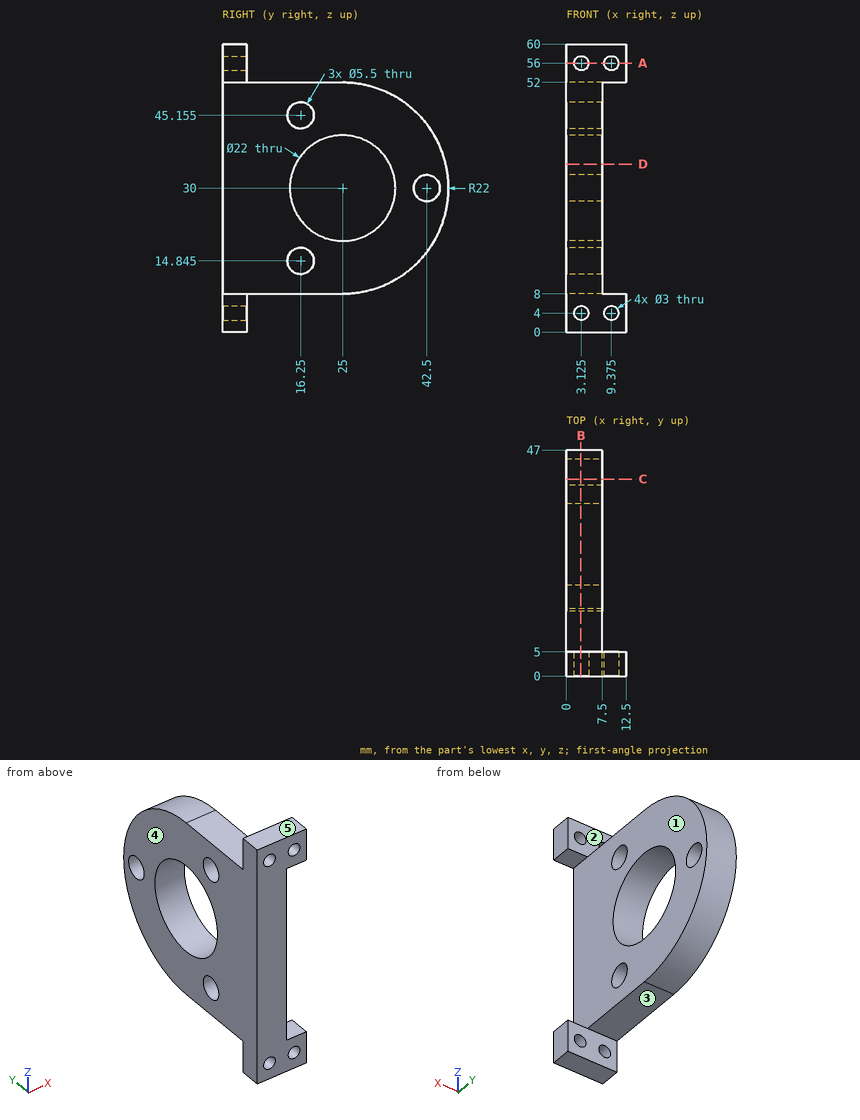
For this review, use the dimensioned drawing (mm, ordinates from the lowest corner) and the shaded views. A direction names the side the tool comes from. Round coordinates to 2 decimals unless told otherwise and drop trailing zeros. Write each loop counter-clockwise with the first axis right and the second up, starting at its lowest first coordinate (ties: lowest second). Pieces come first, ordered by that corner, then holes. Notation, with made-up numbers: M -21,74 L 35,74 A9 cw 35,90 Z; hole C -9,-5 d10. An arc over 180 degrees is marked long. Answer as CSV lines item,"result". Start each with the question number.
Q1. Wall thickness on line 1 along X through (y, z) = (3, 56) (1 decimal); line 2 along Z through (x, y) = (3.5, 16.25) (1 decimal); line 3 along X through (y, z) = (25.5, 43): over which ranges is each line inside the solid? List them lowest first.
Q2. Clearance check with flat-ended pins moving along their axes: P1, Ø5, axis at x = 2.5, y = 12.5, coming from the -Z side; P2, Ø6, axis at x = 8, z = 18, coming from the +Y side; P3, Ø4, axis at x = 4, y = 16, coming from the +Z side. State where each tip first meets the part, or that it passes through.
Q3. Consider section B-B, the plane x = 3. State how many separate pieces and enclosed holes the cut face has, then the cut area to 3 significant figures.
Q4. Tool access review of the marked faces 1, 2, 3, 4 and 5: name each direction out of +Z, -Z, +X, -X, +Y, -Y from which nothing blocks a thin tool from reaching the whole face with its end or side.
Q5. Consider section C-C, the plane y = 41. Give the boundary of the cut face in (x, z) (1 decimal), then the cut area to 3 significant figures.
Q6. Consider section D-D, the plane z = 35. Give the boundary of the cut face in (x, y) (1 decimal).
Q7. Consider section A-A, the plane z = 56. Give the boundary of the cut face in (x, y) (1 decimal).
Result set:
1,line 1,"x = 0 to 1.6, 4.6 to 7.9, 10.9 to 12.5"
1,line 2,"z = 8 to 12.1, 17.6 to 23.3, 36.7 to 42.4, 47.9 to 52"
1,line 3,"x = 0 to 7.5"
2,P1,"stops at z = 8"
2,P2,"stops at y = 45.06"
2,P3,"stops at z = 52"
3,separate pieces,"3"
3,enclosed holes,"4"
3,area,"1,460 mm²"
4,face 1,"+X, +Y, -Y"
4,face 2,"+Z, +X, -X, +Y"
4,face 3,"-Z, +X, -X, +Y"
4,face 4,"+Z, -Z, -X, +Y, -Y"
4,face 5,"+Z, +X, -X, +Y, -Y"
5,outline,"M 0,14.9 L 7.5,14.9 L 7.5,27.7 L 0,27.7 Z; M 0,32.3 L 7.5,32.3 L 7.5,45.1 L 0,45.1 Z"
5,area,"192 mm²"
6,outline,"M 0,0 L 7.5,0 L 7.5,15.2 L 0,15.2 Z; M 0,34.8 L 7.5,34.8 L 7.5,46.4 L 0,46.4 Z"
7,outline,"M 0,0 L 1.6,0 L 1.6,5 L 0,5 Z; M 4.6,0 L 7.9,0 L 7.9,5 L 4.6,5 Z; M 10.9,0 L 12.5,0 L 12.5,5 L 10.9,5 Z"
